Geometry: see drawing. Coordinates: mm, zero at the bounding-box minimum. A direction names the side the tool comes from. Coordinates: 2 decimals unless noted, no trailing zeros. Loops run counter-clockwise (first coordinate to the right, second up) from the corner with the lowest first, then second, coordinate; pieces in that order, holes last. Notation, with made-up numbers: (-5.75, 64) - (33.25, 64) arc R18 ccw to (33.25, 81) - close; hole circle Ø8 at (-25.5, -28.75). An arc over 180 degrees is marked (long way). Use one line per item in the form item = value.
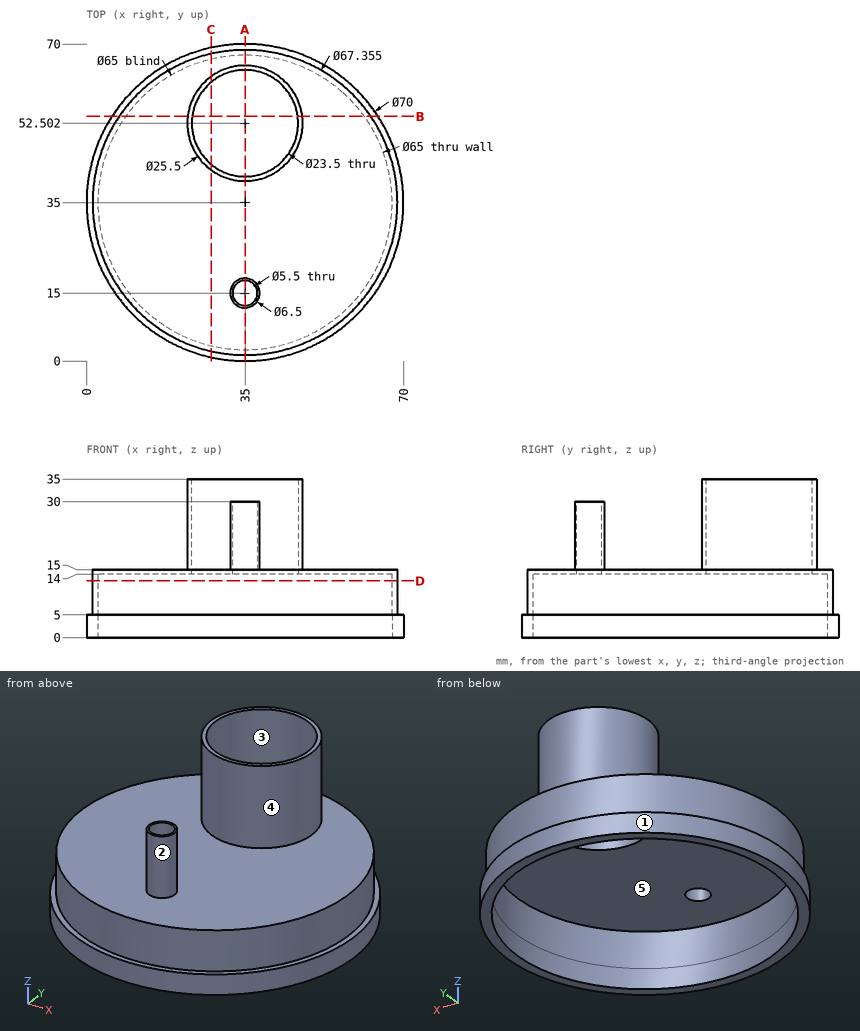
Q1. Pull-direction query (Y, two-part tool) for the marked faces 1 and 2; classes: pulls with the +Y half, pulls with the -Y half, needs draft (parallel to the pull), parting line crosses it, or undercut.
Check values:
face_1 = parting line crosses it
face_2 = undercut
Q2. Cut plane C-C, the plane x = 27.5. Return loops of the section in (y, z).
Check values:
outline = (0.81, 0) - (3.38, 0) - (3.38, 14) - (43.46, 14) - (43.46, 35) - (42.19, 35) - (42.19, 15) - (2.17, 15) - (2.17, 5) - (0.81, 5) - close; (61.55, 14) - (66.62, 14) - (66.62, 0) - (69.19, 0) - (69.19, 5) - (67.83, 5) - (67.83, 15) - (62.81, 15) - (62.81, 35) - (61.55, 35) - close
Q3. Cut plane A-A, the plane x = 35. Return loops of the section in (y, z).
Check values:
outline = (0, 0) - (2.5, 0) - (2.5, 14) - (12.25, 14) - (12.25, 30) - (11.75, 30) - (11.75, 15) - (1.32, 15) - (1.32, 5) - (0, 5) - close; (17.75, 14) - (40.75, 14) - (40.75, 35) - (39.75, 35) - (39.75, 15) - (18.25, 15) - (18.25, 30) - (17.75, 30) - close; (64.25, 14) - (67.5, 14) - (67.5, 0) - (70, 0) - (70, 5) - (68.68, 5) - (68.68, 15) - (65.25, 15) - (65.25, 35) - (64.25, 35) - close
Q4. Cut plane D-D, the plane z = 12.5. Return loops of the section in (x, y) (1 decimal).
Check values:
outline = circle Ø67.4 at (35, 35); hole circle Ø65 at (35, 35)
Q5. First-contact query: P1, Ø3.5, axis at x = 35, y = 15, coming from the -Z side; P2, Ø5, axis at x = 31, z = 11.5, coming from the -Y side; P3, Ø4, axis at y = 39.5, z = 5, coming from the +X side; P4, Ø5, axis at y = 46, z = 9.5, coming from the +X side. Flat tips, straight axial feed; report the tip coordinate or a pass-through.
Check values:
P1 = through
P2 = 1.36
P3 = 69.91
P4 = 67.59
Q6. Set-up query: the marked faces 3, 4 and 5. Return all of +Z, -Z, +X, -X, +Y, -Y with unobstructed straight access to the full face (end or side cutting, diameter ignored); none if empty.
Check values:
face_3 = +Z, -Z
face_4 = +Z
face_5 = -Z
Q7. Cut plane B-B, the plane y = 54. Return loops of the section in (x, z).
Check values:
outline = (5.61, 0) - (8.63, 0) - (8.63, 14) - (23.35, 14) - (23.35, 35) - (22.34, 35) - (22.34, 15) - (7.19, 15) - (7.19, 5) - (5.61, 5) - close; (46.65, 14) - (61.37, 14) - (61.37, 0) - (64.39, 0) - (64.39, 5) - (62.81, 5) - (62.81, 15) - (47.66, 15) - (47.66, 35) - (46.65, 35) - close
Q8. Ray query, line 1 along X through (y, z) = (35, 1.45); line 2 along Z through (x, y) = (45, 15); line 3 along X through (y, z) = (57.5, 3). Return the intervals inside material, ascending. Write a range as [from, to].
Check values:
line_1 = [0, 2.5], [67.5, 70]
line_2 = [14, 15]
line_3 = [8.19, 11.55], [58.45, 61.81]
